from build123d import *

# Parameters (mm, degrees)
EXTRUDE_1_DEPTH          = 3.5
PATTERN_CIRCULAR_1_COUNT = 3


with BuildPart() as part:
    # Sketch 1 → Extrude 1 (new body, symmetric)
    with BuildSketch(Plane(origin=(0, 0, 0), x_dir=(1, 0, 0), z_dir=(0, 1, 0))):
        Polygon((44.845979262, 25.891838199), (37.549878444, 35.934059454), (-37.549878444, 35.934059454), (-44.845979262, 25.891838199), (-49.89474757, 14.552118915), (-12.344869126, -50.486178369), (0, -51.783676398), (12.344869126, -50.486178369), (49.89474757, 14.552118915), align=None)
        with BuildLine():
            Line((-38.750409265, 22.37255922), (-33.983200298, 28.934059454))
            Line((-33.983200298, 28.934059454), (-7.925919728, 28.934059454))
            ThreePointArc((-7.925919728, 28.934059454), (0, 30), (7.925919728, 28.934059454))
            Line((7.925919728, 28.934059454), (33.983200298, 28.934059454))
            Line((33.983200298, 28.934059454), (38.750409265, 22.37255922))
            Line((38.750409265, 22.37255922), (42.04923067, 14.963285033))
            Line((42.04923067, 14.963285033), (29.020590385, -7.602981894))
            ThreePointArc((29.020590385, -7.602981894), (25.980762114, -15), (21.094670658, -21.331077559))
            Line((21.094670658, -21.331077559), (8.066030373, -43.897344487))
            Line((8.066030373, -43.897344487), (0, -44.745118441))
            Line((0, -44.745118441), (-8.066030373, -43.897344487))
            Line((-8.066030373, -43.897344487), (-21.094670658, -21.331077559))
            ThreePointArc((-21.094670658, -21.331077559), (-25.980762114, -15), (-29.020590385, -7.602981894))
            Line((-29.020590385, -7.602981894), (-42.04923067, 14.963285033))
            Line((-42.04923067, 14.963285033), (-38.750409265, 22.37255922))
        make_face(mode=Mode.SUBTRACT)
    extrude(amount=EXTRUDE_1_DEPTH, both=True)

    # Sketch 1_3 → Cut-Revolve 1 (revolve, cut)
    with BuildSketch(Plane(origin=(0, 0, 0), x_dir=(1, 0, 0), z_dir=(0, 1, 0))):
        Polygon((-41.26287783, 16.72946243), (-40.652772865, 18.099780617), (-47.047591069, 20.946937118), (-47.657696033, 19.576618932), align=None)
    cut_revolve_1 = revolve(axis=Axis((0, 0, 0), (-0.913545458, 0, -0.406736643)), mode=Mode.SUBTRACT)

    # Sketch 1_4 → Cut-Revolve 2 (revolve, cut)
    with BuildSketch(Plane(origin=(0, 0, 0), x_dir=(1, 0, 0), z_dir=(0, 1, 0))):
        Polygon((-41.66437521, 30.270940493), (-36.00125625, 26.156443727), (-35.119578371, 27.369969219), (-40.782697332, 31.484465985), align=None)
    cut_revolve_2 = revolve(axis=Axis((0, 0, 0), (-0.809016994, 0, -0.587785252)), mode=Mode.SUBTRACT)

    # Pattern Circular 1: Cut-Revolve 1, Cut-Revolve 2 ×3 about axis
    pattern_circular_1_axis = Axis((0, 3.5, 0), (0, -1, 0))
    for i in range(1, PATTERN_CIRCULAR_1_COUNT):
        add(cut_revolve_1.rotate(pattern_circular_1_axis, i * 360 / PATTERN_CIRCULAR_1_COUNT), mode=Mode.SUBTRACT)
        add(cut_revolve_2.rotate(pattern_circular_1_axis, i * 360 / PATTERN_CIRCULAR_1_COUNT), mode=Mode.SUBTRACT)


solid = part.part
CAD build for the part. Positions are in the model's coordinates, mm. A direction names the side the tool comes from. Round coordinates to 2 decimals unless told otherwise and drop trailing zeros. Loops run counter-clockwise (first coordinate to the right, second up) from the corner with the lowest first, then second, coordinate; pieces in that order, holes last. Notation, with made-up numbers: M -11.5,-17.75 L 2.5,-17.75 A29 cw 2.5,14.25 Z; hole C 3.5,5 d4. An arc over 180 degrees is marked long. One line per question, with ' | ' between items. Start each with the question number.
Item 1: Cut at B-B, the plane z = -1.5. Write the cut outline in (x, y), plus the area to 3 significant figures.
Item 2: Cut at A-A, the plane x = -14. Write the cut outline in (y, z), plus the area to 3 significant figures.
Item 3: Which spindle directions (+Z, -Z, +X, -X, +Y, -Y) get a long thin tool onto all of the face, cutting with end or side? Do faces 4 (the flat face through (7.46, 0.05, 51)), 5 (the flat face through (35.626, 0.049, -3.838)). Say none if no direction does.
Item 4: Wall check: line 1 (X direction, y = 0.25, z = 31); line 2 (Z direction, x = 3.5, y = 3); line 3 (X direction, y = 2.25, z = 38). Give the ranges that are in metal, low to high.
Item 5: Pin check, flat tips, straight feed: pin 1 Ø1.5 at (x, y) = (-22.5, 0.5) entering from +Z; pin 2 Ø3.5 at (x, y) = (-22, 1.5) entering from +Z; pin 3 Ø2 at (y, z) = (2.5, 36.5) entering from +X. Stop position of each tip, or through.
Item 6: Two-plate mould, pull along X, no slides. Class faces 1 (the flat face through (-35.444, 0.049, -3.522)), 2 (the flat face through (-7.63, 0.05, 50.98)), 3 (the flat face through (40.438, 0.049, -31.958)): pulls with the +X half, pulls with the -X half, needs draft (parallel to the pull), parting line crosses it, or undercut.
Responses:
1) outline: M -42.36,-3.5 L -34.28,-3.5 L -34.28,3.5 L -42.36,3.5 Z; M 34.28,-3.5 L 42.36,-3.5 L 42.36,3.5 L 34.28,3.5 Z | area: 113 mm²
2) outline: M -3.5,-35.93 L 3.5,-35.93 L 3.5,-28.93 L -3.5,-28.93 Z; M -3.5,33.62 L 3.5,33.62 L 3.5,47.62 L -3.5,47.62 Z | area: 147 mm²
3) face 4: +Z, +X, +Y, -Y | face 5: +Y, -Y
4) line 1: x = -23.6 to -15.51, 15.51 to 23.6 | line 2: z = -35.93 to -29.8, 44.38 to 51.42 | line 3: x = -19.55 to -11.47, 11.47 to 19.55
5) pin 1: stops at z = 34.2 | pin 2: stops at z = 36.79 | pin 3: stops at x = 21
6) face 1: undercut | face 2: pulls with the -X half | face 3: pulls with the +X half
